from build123d import *

# Parameters (mm, degrees)
SKETCH1_W                        = 66.8528
SKETCH1_H                        = 11.43
BOSS_EXTRUDE1_DEPTH              = 3.175
SKETCH2_W                        = 66.8528
SKETCH2_H                        = 3.175
BOSS_EXTRUDE2_DEPTH              = 93.7514
TAPPED_HOLE_FOR_4_40_HELICOIL1_D = 3.048
LPATTERN1_COUNT                  = 3
LPATTERN1_PITCH                  = 25.4
LPATTERN1_COUNT_DIR2             = 4
LPATTERN1_PITCH_DIR2             = 25.4
F_30_0_1285_DIAMETER_HOLE1_D     = 3.2639
RIB3_REACH                       = 109.949
SKETCH15_WALL_W                  = 244.822615678
SKETCH15_WALL_H                  = 2.54
RIB4_REACH                       = 109.949
SKETCH16_WALL_W                  = 244.822615678
SKETCH16_WALL_H                  = 2.54
TAPPED_HOLE_FOR_4_40_HELICOIL3_D = 3.048
FILLET1_R                        = 2.54
TAPPED_HOLE_FOR_4_40_HELICOIL4_D = 3.048


with BuildPart() as part:
    # Sketch1 → Boss-Extrude1 (new body)
    with BuildSketch(Plane(origin=(0, 0, 0), x_dir=(1, 0, 0), z_dir=(0, 1, 0))):
        with Locations((33.4264, 5.715)):
            Rectangle(SKETCH1_W, SKETCH1_H)
    extrude(amount=BOSS_EXTRUDE1_DEPTH)

    # Sketch2 → Boss-Extrude2 (add)
    with BuildSketch(Plane(origin=(0, 3.175, 0), x_dir=(1, 0, 0), z_dir=(0, 1, 0))):
        with Locations((33.4264, 1.5875)):
            Rectangle(SKETCH2_W, SKETCH2_H)
    extrude(amount=BOSS_EXTRUDE2_DEPTH)

    # Tapped Hole for #4-40 Helicoil1 (through all)
    with Locations(Plane.XY):
        with Locations((8.0264, 88.9)):
            tapped_hole_for_4_40_helicoil1 = Hole(TAPPED_HOLE_FOR_4_40_HELICOIL1_D / 2)

    # LPattern1: Tapped Hole for _4-40 Helicoil1 3 × 4
    with Locations(*[(i * LPATTERN1_PITCH, -j * LPATTERN1_PITCH_DIR2, 0) for i in range(LPATTERN1_COUNT) for j in range(LPATTERN1_COUNT_DIR2) if (i, j) != (0, 0)]):
        add(tapped_hole_for_4_40_helicoil1, mode=Mode.SUBTRACT)

    # #30 (0.1285) Diameter Hole1 (through all)
    with Locations(Plane(origin=(0, 3.175, 0), x_dir=(1, 0, 0), z_dir=(0, 1, 0))):
        with Locations((8.0264, 8.001), (33.4264, 8.001), (58.8264, 8.001)):
            Hole(F_30_0_1285_DIAMETER_HOLE1_D / 2)

    # Sketch15 wall → Rib3 (add, up to next)
    with BuildSketch(Plane(origin=(46.1264, 15.988809865, -7.3025), x_dir=(0, 0.951838472973, 0.306599937001), z_dir=(0, 0.306599937001, -0.951838472973)), mode=Mode.PRIVATE) as rib3_sk1:
        Rectangle(SKETCH15_WALL_W, SKETCH15_WALL_H)
    rib3_tool1 = extrude(rib3_sk1.sketch, amount=-RIB3_REACH, mode=Mode.PRIVATE) - part.part
    add(rib3_tool1.solids().sort_by_distance((46.1264, 15.988809865, -7.3025))[0])

    # Sketch16 wall → Rib4 (add, up to next)
    with BuildSketch(Plane(origin=(20.7264, 15.988809865, -7.3025), x_dir=(0, 0.951838472973, 0.306599937001), z_dir=(0, 0.306599937001, -0.951838472973)), mode=Mode.PRIVATE) as rib4_sk1:
        Rectangle(SKETCH16_WALL_W, SKETCH16_WALL_H)
    rib4_tool1 = extrude(rib4_sk1.sketch, amount=-RIB4_REACH, mode=Mode.PRIVATE) - part.part
    add(rib4_tool1.solids().sort_by_distance((20.7264, 15.988809865, -7.3025))[0])

    # Tapped Hole for #4-40 Helicoil3 (through all)
    with Locations(Plane.XY):
        with Locations((27.0764, 56.515), (39.7764, 56.515), (33.4264, 82.169), (20.7264, 63.5), (46.1264, 63.5)):
            Hole(TAPPED_HOLE_FOR_4_40_HELICOIL3_D / 2)

    # Fillet1
    fillet1_edges = [part.edges().sort_by_distance(p)[0] for p in [
        (21.9964, 15.988809865, -3.175),
        (19.4564, 15.988809865, -3.175),
        (66.8528, 96.9264, -1.5875),
        (0, 96.9264, -1.5875),
        (0, 1.5875, -11.43),
        (66.8528, 1.5875, -11.43),
        (47.3964, 15.988809865, -3.175),
        (44.8564, 15.988809865, -3.175),
    ]]
    fillet(fillet1_edges, radius=FILLET1_R)

    # Tapped Hole for #4-40 Helicoil4 (through all)
    with Locations(Plane.XY):
        with Locations((3.4264, 93.5), (3.4264, 33.5), (63.4264, 33.5), (63.4264, 93.5), (18.4264, 78.5), (48.4264, 78.5), (48.4264, 48.5), (18.4264, 48.5)):
            Hole(TAPPED_HOLE_FOR_4_40_HELICOIL4_D / 2)


solid = part.part
The model under review builds one solid part; all positions refer to its coordinate system, in mm. A direction names the side the tool comes from. Round coordinates to 2 decimals unless told otherwise and drop trailing zeros. Write each loop counter-clockwise with the first axis right and the second up, starting at its lowest first coordinate (ties: lowest second). Pieces come first, ordered by that corner, then holes. Notation, with made-up numbers: (-2, 47.5) - (34, 47.5) arc R22 cw to (34, 59.5) - close; hole circle Ø8 at (2, 29.25). An arc over 180 degrees is marked (long way). One line per item, written item: value. Start each with the question number.
1. Clearance check with flat-ended pins moving along their axes: P1, Ø1.5, axis at x = 10, z = -9, coming from the -Y side; P2, Ø4.5, axis at y = 13.5, z = -9.5, coming from the +X side; P3, Ø10, axis at x = 50, y = 79.5, coming from the -Z side (3 decimals); P4, Ø4, axis at x = 36, z = -6, coming from the +Y side (3 decimals). State where each tip first meets the part, or that it passes through.
2. Consider section B-B on x = 33. State how many separate pieces and enclosed holes the cut face has, and give its area (3 significant figures).
3. Consider section D-D on x = 21. Write out the cut boundary in (y, z) (3 decimals), and give its area (3 significant figures).
4. To check wall thickness, follow L1, parallel to X at y = 5.5, z = -10.5; L2, parallel to Y at x = 19.5, z = -1.5; L3, parallel to X at y = 33, z = -2.75. State the ranges of each line that lie inside material, in increasing order. Write a range as from..to.
5. Consider section A-A on y = 38.1. Write out the cut boundary in (x, z) (3 decimals), and give its area (3 significant figures).
6. The part is to be moulded in two halves that separate along Y. For faces 4 (the face through (48.62, 80.01, -1.61)), 5 (the face through (8.38, 1.565, -6.408)), say which applies: released by +Y, released by -Y, zero draft, split by the parting line, or undercut.
7. Machinability: for faces 1 (the face through (19.456, 9, -8)), 2 (the face through (33.62, 65.01, -1.61)), 3 (the face through (44.856, 9, -8)), which of the approach directions +Z, -Z, +X, -X, +Y, -Y give a long, thin tool a straight path to every point of the face, cutting with its end or side? Answer none if there is none.
Checks:
1. P1: stops at y = 0
1. P2: stops at x = 47.4
1. P3: stops at z = -3.175
1. P4: stops at y = 3.175
2. separate pieces: 7
2. enclosed holes: 0
2. area: 277 mm^2
3. outline: (0, -11.43) - (3.175, -11.43) - (28.803, -3.175) - (62.001, -3.175) - (62.001, 0) - (0, 0) - close; (64.999, -3.175) - (96.926, -3.175) - (96.926, 0) - (64.999, 0) - close
3. area: 430 mm^2
4. L1: x = 19.46..22, 44.86..47.4
4. L2: y = 0..47.42, 49.58..62.6, 64.4..77.42, 79.58..96.93
4. L3: x = 0..1.99, 4.87..61.99, 64.87..66.85
5. outline: (0, -3.175) - (6.502, -3.175) - (6.502, 0) - (0, 0) - close; (9.55, -3.175) - (31.902, -3.175) - (31.902, 0) - (9.55, 0) - close; (34.95, -3.175) - (57.302, -3.175) - (57.302, 0) - (34.95, 0) - close; (60.35, -3.175) - (66.853, -3.175) - (66.853, 0) - (60.35, 0) - close
5. area: 183 mm^2
6. face 4: undercut
6. face 5: zero draft
7. face 1: -Z, -X, +Y
7. face 2: +Z, -Z
7. face 3: -Z, +Y
